The listing builds one solid part. Answer for the finished solid, in the listing's coordinates (mm). Coordinates: 2 decimals unless noted, no trailing zeros. Loops run counter-clockwise (first coordinate to the right, second up) from the corner with the lowest first, then second, coordinate; pieces in that order, holes last. Notation, with made-up numbers: (11, 53) - (49, 53) arc R9 cw to (49, 59) - close; hole circle Ø4 at (73.5, 34). An arc over 180 degrees is marked (long way). Use one line per item in the form item = value. Start each with the question number.
```python
from build123d import *

# Parameters (mm, degrees)
F1_DEPTH      = 700
F2_R          = 100
F3_DEPTH      = 400
F3_DEPTH_BACK = 310


with BuildPart() as f1:
    # F0 (on Front) → F1 (new body)
    with BuildSketch(Plane.XZ):
        Polygon((270.7016063785, -167.6180982615), (124.1205126206, 332.3819017385), (-125.8794873794, 332.3819017385), (-229.2983936215, -167.6180982615), align=None)
    extrude(amount=-F1_DEPTH)

    # F2 (on Right) → F3 (cut, two sides)
    with BuildSketch(Plane.YZ) as f3_sk:
        with Locations((200, 332.3819017385)):
            Circle(F2_R)
        with Locations((500, 332.3819017385)):
            Circle(F2_R)
    extrude(amount=-F3_DEPTH, mode=Mode.SUBTRACT)
    extrude(f3_sk.sketch, amount=F3_DEPTH_BACK, mode=Mode.SUBTRACT)


solid = f1.part
```
(1) A cutting plane is placed at C-C (z = 163). Determine the outline of the cut face in (x, y).
(2) A cutting plane is placed at B-B (y = 200). Determine the outline of the cut face in (x, z), then the cut area to 3 significant figures.
(3) Find the intervals of material crossed by probe 1 along Y at (x, z) = (-51.5, 300); probe 2 along Z at (x, y) = (106, 199.5); probe 3 along Z at (x, y) = (-133.5, 195), in increasing order. Write a range as from..to.
(4) A cutting plane is placed at A-A (x = 101). Determine the outline of the cut face in (y, z), then the cut area to 3 significant figures.
(5) Each of these flat-tipped pins is pushed along its axis until it touches: pin 1 Ø5 at (y, z) = (248.5, 236) entering from -X; pin 2 Ø8 at (y, z) = (549, 46.5) entering from -X; pin 3 Ø10 at (x, y) = (68.5, 445.5) entering from +Z. Where does it stop, or does it pass through?
Evaluation:
q1.outline = (-160.91, 0) - (173.78, 0) - (173.78, 700) - (-160.91, 700) - close
q2.outline = (-229.3, -167.62) - (270.7, -167.62) - (153.44, 232.38) - (-146.56, 232.38) - close
q2.area = 160,000 mm^2
q3.probe_1 = 0..105.39, 294.61..405.39, 594.61..700
q3.probe_2 = -167.62..232.38
q3.probe_3 = -167.62..232.51
q4.outline = (0, -167.62) - (700, -167.62) - (700, 332.38) - (600, 332.38) arc R100 cw to (400, 332.38) - (300, 332.38) arc R100 cw to (100, 332.38) - (0, 332.38) - close
q4.area = 319,000 mm^2
q5.pin_1 = -146.33
q5.pin_2 = -185.84
q5.pin_3 = 252.01
